Autodesk Fusion 360 part; units mm, degrees
sketch "Sketch1" plane through (0, 0, 0) normal (0, 0, 1) x (1, 0, 0)
  line L0 (0, 0) -> (36, 0)
  line L1 (36, 0) -> (36, 18)
  line L2 (36, 18) -> (0, 18)
  line L3 (0, 18) -> (0, 0)
  dimension "d1" = 36
  dimension "d2" = 18
extrude "Extrude1" add sketch "Sketch1" along normal blind 20
sketch "Sketch2" plane through (0, 0, 20) normal (0, 0, 1) x (-1, 0, 0)
  line L0 (0, -18) -> (0, 0)
  line L1 (0, 0) -> (-36, 0)
  line L2 (-36, 0) -> (-36, -18)
  line L3 (-36, -18) -> (0, -18)
  circle A0 centre (-18, -18) radius 13
  dimension "d5" = 26
extrude "Extrude2" cut sketch "Sketch2" against normal blind 20 contours L3 A0 picked at (-19.0768, -11.2377)
ref_plane "WorkPlane1" through (0, 20, 0) normal (0, 1, 0) x (0, 0, 1)
sketch "Sketch7" plane through (0, 0, 0) normal (0, -1, 0) x (1, 0, 0)
  line L0 (0, 0) -> (36, 0)
  line L1 (36, 20) -> (0, 20)
  line L2 (0, 20) -> (0, 0)
  line L3 (18, 10) -> (18, 23) construction
  line L4 (36, 0) -> (36, 20)
sketch "Sketch6" plane through (36, 0, 0) normal (1, 0, 0) x (0, 1, 0)
  line L0 (0, 0) -> (18, 0)
  line L1 (18, 0) -> (18, 20)
  line L2 (18, 20) -> (0, 20)
  line L3 (0, 20) -> (0, 0)
  line L4 (0, 20) -> (18, 0) construction
  line L5 (0, 0) -> (18, 20) construction
  line L6 (9, 10) -> (18, 10) construction
  line L7 (9, 10) -> (9, 0) construction
  line L8 (9, 10) -> (9, 20) construction
  line L9 (13.5, 17.5) -> (18, 17.5) construction
  line L10 (13.5, 5) -> (13.5, 10) construction
  line L11 (18, 7.5) -> (18, 12.5311)
  line L12 (13.5, 17.5) -> (18, 17.5)
  line L13 (18, 17.5) -> (18, 2.5)
  line L14 (18, 2.5) -> (13.5, 2.5)
  line L15 (13.5, 2.5) -> (13.5, 17.5)
  dimension "d25" = 15
  dimension "d26" = 4.5
  dimension "d34" = 7.5
extrude "Extrude7" add sketch "Sketch6" along normal blind 8 contours L1 L11 L12 L13 L14 L15
sketch "Sketch11" plane through (0, 13.5, 0) normal (0, -1, 0) x (1, 0, 0)
  line L0 (36, 17.5) -> (36, 2.5)
  line L1 (36, 2.5) -> (44, 2.5)
  line L2 (44, 2.5) -> (44, 17.5)
  line L3 (44, 17.5) -> (36, 17.5)
  circle A0 centre (40, 13) radius 1.1
  circle A1 centre (40, 7) radius 1.1
  line L4 (36, 0) -> (36, 20)
  line L5 (36, 20) -> (0, 20)
  line L6 (18, 10) -> (18, 23)
  circle A2 centre (-4, 13) radius 1.1
  circle A3 centre (-4, 7) radius 1.1
  dimension "d30" = 2.2
  dimension "d31" = 2.2
  dimension "d35" = 6
  dimension "d36" = 4
  dimension "d37" = 4
  dimension "d38" = 7
sketch "Sketch12" plane through (0, 0, 0) normal (-1, 0, 0) x (0, -1, 0)
  line L0 (-18, 0) -> (0, 0)
  line L1 (0, 0) -> (0, 20)
  line L2 (0, 20) -> (-18, 20)
  line L3 (-18, 20) -> (-18, 0)
  line L4 (-18, 17.5) -> (-13.5, 17.5)
  line L5 (-13.5, 17.5) -> (-13.5, 2.5)
  line L6 (-13.5, 2.5) -> (-18, 2.5)
  line L7 (-18, 2.5) -> (-18, 17.5)
  line L8 (-18, 10) -> (-8, 10) construction
  dimension "d39" = 15
  dimension "d40" = 7.5
  dimension "d41" = 4.5
extrude "Extrude8" add sketch "Sketch12" along normal blind 8 contours L3 L4 L5 L6 L7
extrude "Extrude9" cut sketch "Sketch11" against normal blind 4.5 contours A0 | A1 | A2 | A3
fillet "Fillet4" radius 0.5 1 edges at (0, 13.5, 10)
fillet "Fillet5" radius 1 2 edges at (-8, 18, 10) (-8, 13.5, 10)
fillet "Fillet6" radius 1 2 edges at (44, 13.5, 10) (44, 18, 10)
fillet "Fillet7" radius 0.5 1 edges at (36, 13.5, 10)
fillet "Fillet9" radius 12 2 edges at (36, 0, 10) (0, 0, 10)
The model under review builds one solid part; all positions refer to its coordinate system, in mm. A direction names the side the tool comes from. Round coordinates to 2 decimals unless told otherwise and drop trailing zeros. Write each loop counter-clockwise with the first axis right and the second up, starting at its lowest first coordinate (ties: lowest second). Pieces come first, ordered by that corner, then holes. Notation, with made-up numbers: (57.5, 21) -> (73.5, 21) arc R25 ccw to (73.5, 37) -> close; hole circle Ø5 at (-36.75, 73.5). An arc over 180 degrees is marked (long way). Use CSV: the item, a comma, the result in double quotes.
Q1. Mouldability with a two-part tool opening along X and no side actions: class faces 5 (the cylindrical face through (43.699, 13.785, 10.105)), 6 (the flat face through (-4, 13.5, 10)), 7 (the cylindrical face through (40.508, 15.718, 12.024)) as released by +X, released by -X, zero draft, split by the parting line, or undercut.
Checks:
face 5,"released by +X"
face 6,"zero draft"
face 7,"undercut"
Q2. For faces 1 (the flat face through (-4, 16, 2.5)), 2 (the flat face through (40, 16, 17.5)), 3 (the flat face through (40, 16, 2.5)), 4 (the flat face through (-4, 16, 17.5)), list the 3-axis set-ups (+Z, -Z, +X, -X, +Y, -Y) from which the entire face can be reached by the end or side of a thin tool; tool diameter is ignored.
Checks:
face 1,"-Z, -X, +Y, -Y"
face 2,"+Z, +X, +Y, -Y"
face 3,"-Z, +X, +Y, -Y"
face 4,"+Z, -X, +Y, -Y"
Q3. For pin 1 Ø7 at (x, z) = (-4.5, 6.5) entering from -Y; pin 2 Ø4 at (x, y) = (40.5, 16) entering from -Z; pin 3 Ø2 at (x, z) = (40, 13) entering from -Y; pin 4 Ø2.5 at (x, y) = (-6, 16.5) entering from +Z, all flat-tipped, find the tip position at first contact; note any pin that passes through.
Checks:
pin 1,"y = 13.5"
pin 2,"z = 2.5"
pin 3,"through"
pin 4,"z = 17.5"
Q4. Consider section C-C (z = 13). Give the boundary of the cut face in (x, y), then the cut area to 3 significant figures.
Checks:
outline,"(-8, 14.5) arc R1 ccw to (-7, 13.5) -> (-5.1, 13.5) -> (-5.1, 18) -> (-7, 18) arc R1 ccw to (-8, 17) -> close; (-2.9, 13.5) -> (-0.5, 13.5) arc R0.5 cw to (0, 13) -> (0, 12) arc R12 ccw to (12, 0) -> (24, 0) arc R12 ccw to (36, 12) -> (36, 13) arc R0.5 cw to (36.5, 13.5) -> (38.9, 13.5) -> (38.9, 18) -> (31, 18) arc R13 cw to (5, 18) -> (-2.9, 18) -> close; (41.1, 13.5) -> (43, 13.5) arc R1 ccw to (44, 14.5) -> (44, 17) arc R1 ccw to (43, 18) -> (41.1, 18) -> close"
area,"372 mm²"
Q5. Consider section B-B (y = 15.25). Give the boundary of the cut face in (x, z).
Checks:
outline,"(-8, 2.5) -> (0, 2.5) -> (0, 0) -> (5.29, 0) -> (5.29, 20) -> (0, 20) -> (0, 17.5) -> (-8, 17.5) -> close; (30.71, 0) -> (36, 0) -> (36, 2.5) -> (44, 2.5) -> (44, 17.5) -> (36, 17.5) -> (36, 20) -> (30.71, 20) -> close; hole circle Ø2.2 at (-4, 7); hole circle Ø2.2 at (-4, 13); hole circle Ø2.2 at (40, 7); hole circle Ø2.2 at (40, 13)"
Q6. To check wall thickness, follow probe 1 along Z at (x, y) = (-4, 14.8); probe 2 along X at (y, z) = (17, 18.75); probe 3 along Y at (x, z) = (18.5, 15.5). State the ranges of each line that lie inside material, in increasing order. Write a range as [from, to].
Checks:
probe 1,"[2.5, 5.9], [8.1, 11.9], [14.1, 17.5]"
probe 2,"[0, 5.04], [30.96, 36]"
probe 3,"[0, 5.01]"
Q7. Consider section D-D (y = 11.5). Give the boundary of the cut face in (x, z), then the cut area to 3 significant figures.
Checks:
outline,"(0.01, 0) -> (6.74, 0) -> (6.74, 20) -> (0.01, 20) -> close; (29.26, 0) -> (35.99, 0) -> (35.99, 20) -> (29.26, 20) -> close"
area,"269 mm²"
Q8. Consider section A-A (x = -4). Give the boundary of the cut face in (y, z).
Checks:
outline,"(13.5, 2.5) -> (18, 2.5) -> (18, 5.9) -> (13.5, 5.9) -> close; (13.5, 8.1) -> (18, 8.1) -> (18, 11.9) -> (13.5, 11.9) -> close; (13.5, 14.1) -> (18, 14.1) -> (18, 17.5) -> (13.5, 17.5) -> close"
